Here's how the part is built. I have some questions about the finished solid (model axes, mm). Face numbers are marked on the shaded views. A direction names the side the tool comes from. Coordinates: 2 decimals unless noted, no trailing zeros. Write each loop counter-clockwise with the first axis right and the second up, starting at its lowest first coordinate (ties: lowest second). Pieces come first, ordered by that corner, then holes.
(1) For pin 1 Ø5 at (x, z) = (-8.5, 14) entering from -Y; pin 2 Ø25 at (x, y) = (0, 0) entering from +Z; pin 3 Ø2 at (y, z) = (-12, 14) entering from +X, each with a flat end and sliding along its axis, tell me the tip position at first contact or that it passes through.
(2) Which directions (+Z, -Z, +X, -X, +Y, -Y) give clear straight access to the entire face, cutting with the end or side of a thin tool? Please do the marked faces 1, 2, 3 and 4.
(3) Imagine slicing it at D-D, the plane y = 17.5. List the corners of the cut face in (x, z) for me, plus the area to 3 significant figures.
(4) Thinking about a two-plate mould opening in X: for the marked faces 5, 6, 7 and 8, which applies, released by +X, released by -X, zero draft, split by the parting line, or undercut?
(5) Imagine slicing it at B-B, the plane x = -3.5. List the corners of the cut face in (y, z) for me.
(6) Imagine slicing it at C-C, the plane x = -11.5. List the corners of the cut face in (y, z) for me, plus the area to 3 significant figures.
(7) Please list where these lines run through material, in increasing order: probe 1 along Z at (x, y) = (4.5, 17); probe 2 along X at (y, z) = (0, 13.5); probe 3 along Y at (x, z) = (-11.5, 9.75).
(8) Imagine slicing it at A-A, the plane z = 2.5. List the corners of the cut face in (x, y) for me.
Autodesk Inventor part; units mm, degrees
ref_plane "YZ Plane" through (0, 0, 0) normal (1, 0, 0) x (0, 1, 0)
ref_plane "XZ Plane" through (0, 0, 0) normal (0, 1, 0) x (-1, 0, 0)
ref_plane "XY Plane" through (0, 0, 0) normal (0, 0, 1) x (1, 0, 0)
sketch "Sketch1" plane through (0, 0, 0) normal (0, 0, 1) x (1, 0, 0)
  circle A0 centre (0, 0) radius 15.75
  circle A1 centre (0, 0) radius 21.75
  dimension "d1" = 31.5
  dimension "d2" = 43.5
extrude "Extrusion1" add sketch "Sketch1" along normal blind 6.35 contours A0 | A1
sketch "Sketch2" plane through (0, 0, 6.35) normal (0, 0, 1) x (1, 0, 0)
  circle A0 centre (0, 0) radius 21.75
  circle A1 centre (0, 0) radius 15.75
  dimension "d5" = 31.5
extrude "Extrusion2" add sketch "Sketch2" along normal blind 6.35
sketch "Sketch3" plane through (0, 0, 6.35) normal (0, 0, 1) x (1, 0, 0)
  line L0 (0, -4.75) -> (0, -8.25)
  line L1 (0, -8.25) -> (0, -4.75)
  line L2 (0, 4.75) -> (0, 8.25)
  line L3 (0, 0) -> (0, -1.75)
  line L4 (0, 0) -> (0, 1.75)
  line L5 (0, 0) -> (0, 2.25)
  line L6 (0, 0) -> (0, -2.25)
  line L7 (4.7631, 0) -> (0, 0)
  arc A0 (-5.5, -2.25) -> (5.5, -2.25) centre (0, -2.25) ccw
  arc A1 (5.5, 2.25) -> (-5.5, 2.25) centre (0, 2.25) ccw
  line L8 (-5.5, 2.25) -> (-5.5, -2.25)
  line L9 (5.5, 2.25) -> (5.5, -2.25)
  point P0 (-5.5102, 0)
  dimension "d11" = 8.25
  dimension "d12" = 8.25
  dimension "d32" = 2.25
  dimension "d33" = 2.25
extrude "Extrusion3" cut sketch "Sketch3" along normal through all both and the other way through all
sketch "Sketch4" plane through (0, 0, 12.7) normal (0, 0, 1) x (1, 0, 0)
  point P0 (0, 0)
sketch "Sketch5" plane through (0, 0, 12.7) normal (0, 0, 1) x (1, 0, 0)
  circle A0 centre (0, 0) radius 15.75
  line L0 (0, 15.75) -> (0, 21.75)
  circle A1 centre (0, 0) radius 21.75
  line L1 (-14.7967, 5.3964) -> (-20.2679, 7.8914)
  arc A2 (0, 15.75) -> (-14.7967, 5.3964) centre (0, 0) ccw
  arc A3 (0, 21.75) -> (-20.2679, 7.8914) centre (0, 0) ccw
extrude "Extrusion4" cut sketch "Sketch5" against normal blind 6.35 contours A0 L1 A1 L0 picked at (-1.7226, 19.5424)
sketch "Sketch6" plane through (0, 0, 12.7) normal (0, 0, 1) x (1, 0, 0)
  point P0 (0, 0)
sketch "Sketch7" plane through (0, 0, 12.7) normal (0, 0, 1) x (1, 0, 0)
  circle A0 centre (0, 0) radius 21.75
  circle A1 centre (0, 0) radius 15.75
extrude "Extrusion5" add sketch "Sketch7" against normal blind 6.35
sketch "Sketch8" plane through (0, 0, 12.7) normal (0, 0, 1) x (1, 0, 0)
  point P0 (0, 0)
sketch "Sketch9" plane through (0, 0, 12.7) normal (0, 0, 1) x (1, 0, 0)
  circle A0 centre (0, 0) radius 15.75
  circle A1 centre (0, 0) radius 21.75
  circle A2 centre (0, 0) radius 21.75
  circle A3 centre (0, 0) radius 15.75
  line L0 (15.7497, -0.1038) -> (21.6454, 2.1307)
  arc A4 (15.7497, -0.1038) -> (0, 15.75) centre (0, 0) ccw
  arc A5 (21.6454, 2.1307) -> (2.0753, 21.6508) centre (0, 0) ccw
  line L1 (0, 15.75) -> (0.0466, 21.7499)
  circle A6 centre (0, 0) radius 21.75
  arc A7 (21.6454, 2.1307) -> (0.0466, 21.7499) centre (0, 0) ccw
extrude "Extrusion6" cut sketch "Sketch9" against normal blind 6.35 contours A0 L1 A1 L0 picked at (4.1755, 19.2056)
sketch "Sketch10" plane through (0, 0, 12.7) normal (0, 0, 1) x (1, 0, 0)
  circle A0 centre (0, 0) radius 15.75
  circle A1 centre (0, 0) radius 21.75
  point P0 (15.7497, -0.1038)
extrude "Extrusion7" add sketch "Sketch10" along normal blind 6.35
sketch "Sketch11" plane through (0, 0, 19.05) normal (0, 0, 1) x (1, 0, 0)
  circle A0 centre (0, 0) radius 21.75
  circle A1 centre (0, 0) radius 15.75
  circle A2 centre (0, 0) radius 21.75
  arc A3 (0, 15.75) -> (15.7497, -0.1038) centre (0, 0) ccw
  line L0 (12.1903, -9.9729) -> (16.8342, -13.7721)
  line L1 (-12.1903, 9.9729) -> (-16.8342, 13.7721)
  arc A4 (12.1903, -9.9729) -> (-12.1903, 9.9729) centre (0, 0) ccw
  arc A5 (16.8342, -13.7721) -> (-16.8342, 13.7721) centre (0, 0) ccw
  line L2 (-12.1903, 9.9729) -> (-16.8342, 13.7721)
  line L3 (12.1903, -9.9729) -> (16.8342, -13.7721)
  arc A6 (12.1903, -9.9729) -> (-12.1903, 9.9729) centre (0, 0) ccw
  point P0 (6.5, 1.75)
  point P1 (-6.5, 1.75)
extrude "Extrusion8" cut sketch "Sketch11" against normal blind 6.35 contours A0 L0 A1 L1 picked at (19.4008, 2.9309)
properties part number "bracket"
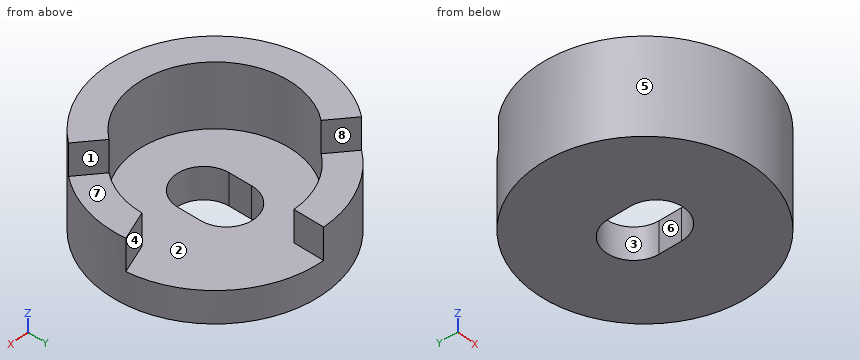
Recorded:
1. pin 1: stops at y = -20.91
1. pin 2: stops at z = 6.35
1. pin 3: stops at x = 15.89
2. face 1: +Z, +X, +Y
2. face 2: +Z
2. face 3: +Z, -Z
2. face 4: +Z, +Y
3. outline: (-12.92, 0) - (12.92, 0) - (12.92, 6.35) - (0.01, 6.35) - (0.01, 12.7) - (-12.92, 12.7) - close
3. area: 246 mm2
4. face 5: split by the parting line
4. face 6: undercut
4. face 7: zero draft
4. face 8: released by +X
5. outline: (-21.47, 0) - (-6.49, 0) - (-6.49, 6.35) - (-15.36, 6.35) - (-15.36, 19.05) - (-21.47, 19.05) - close; (6.49, 0) - (21.47, 0) - (21.47, 12.7) - (15.36, 12.7) - (15.36, 6.35) - (6.49, 6.35) - close
6. outline: (-18.46, 0) - (18.46, 0) - (18.46, 12.7) - (10.76, 12.7) - (10.76, 6.35) - (-10.76, 6.35) - (-10.76, 19.05) - (-18.46, 19.05) - close
6. area: 381 mm2
7. probe 1: z = 0 to 6.35
7. probe 2: x = -21.75 to -15.75
7. probe 3: y = -18.46 to -10.76, 10.76 to 18.46
8. outline: circle Ø43.5 at (0, 0); hole (-5.5, -2.25) arc R5.5 ccw to (5.5, -2.25) - (5.5, 2.25) arc R5.5 ccw to (-5.5, 2.25) - close
